Check sheet for the drawn part. Datum: minimum x, y, z corner. Units: mm. A direction names the side the tool comes from. Round coordinates to 2 decimals unless told otherwise and drop trailing zeros. Loops run counter-clockwise (first coordinate to the right, second up) from the corner with the lowest first, then second, coordinate; pieces in that order, holes last.
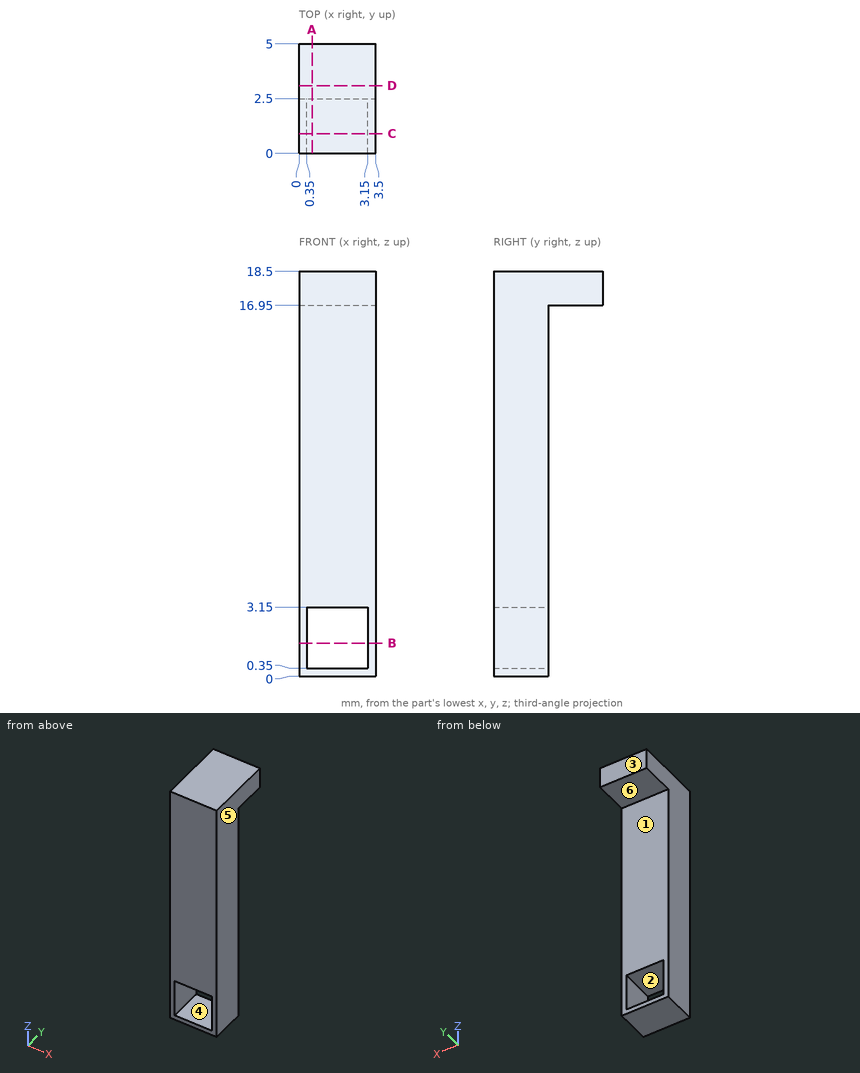
1. Section check C-C (y = 0.9). Enter the section's corners in (x, z).
2. Section check D-D (y = 3.1). Enter the section's corners in (x, z).
3. Section check B-B (z = 1.5). Enter the section's corners in (x, y).
4. Scan lines: L1, parallel to Z at x = 2.6, y = 1; L2, parallel to X at y = 1.55, z = 2; L3, parallel to Z at x = 1.55, y = 3.95. Record each from-to range of solid material in increasing order.
5. Release check for a two-part mould opening along X. For the marked faces 4, 5 and 6 record: released by +X, released by -X, zero draft, split by the parting line, or undercut.
6. Tool access check on the marked faces 1, 2 and 3. Record the directions out of +Z, -Z, +X, -X, +Y, -Y that give a thin tool (end or side, any length) a straight path to the whole face; none if there is none.
7. Gauge pin test, flat ends, axial feed: P1, Ø2, axis at y = 2, z = 1, coming from the -X side; P2, Ø1.8, axis at x = 1.5, z = 9.5, coming from the +Y side. Record the tip position at first contact, or that the pin passes through.
8. Section check A-A (x = 0.6). Enter the section's corners in (y, z), then the cut area to 3 significant figures.
Taken from the geometry:
1. outline: (0, 0) - (3.5, 0) - (3.5, 18.5) - (0, 18.5) - close; hole (0.35, 0.35) - (3.15, 0.35) - (3.15, 3.15) - (0.35, 3.15) - close
2. outline: (0, 16.95) - (3.5, 16.95) - (3.5, 18.5) - (0, 18.5) - close
3. outline: (0, 0) - (0.35, 0) - (0.35, 2.5) - (0, 2.5) - close; (3.15, 0) - (3.5, 0) - (3.5, 2.5) - (3.15, 2.5) - close
4. L1: z = 0 to 0.35, 3.15 to 18.5
4. L2: x = 0 to 0.35, 3.15 to 3.5
4. L3: z = 16.95 to 18.5
5. face 4: undercut
5. face 5: released by +X
5. face 6: zero draft
6. face 1: -Z, +X, -X, +Y
6. face 2: +Y, -Y
6. face 3: +Z, -Z, +X, -X, +Y
7. P1: stops at x = 0
7. P2: stops at y = 2.5
8. outline: (0, 0) - (2.5, 0) - (2.5, 0.35) - (0, 0.35) - close; (0, 3.15) - (2.5, 3.15) - (2.5, 16.95) - (5, 16.95) - (5, 18.5) - (0, 18.5) - close
8. area: 43.1 mm2
